from build123d import *

# Parameters (mm, degrees)
F0_R     = 1.75
F1_DEPTH = 1.5


with BuildPart() as f1:
    # F0 (on Right) → F1 (new body)
    with BuildSketch(Plane.YZ):
        Polygon((-3, -1.5), (-3, 0), (3, 0), (3, -1.5), (8, -1.5), (8, 0), (9, 0), (14.459554, 15), (9, 30), (8, 30), (8, 31.5), (3, 31.5), (3, 30), (-3, 30), (-3, 31.5), (-8, 31.5), (-8, 30), (-9, 30), (-3.540446, 15), (-9, 0), (-8, 0), (-8, -1.5), align=None)
        with Locations((0.459554, 15)):
            Circle(F0_R, mode=Mode.SUBTRACT)
    extrude(amount=F1_DEPTH)


solid = f1.part
Geometry: final body of the model. Coordinates: model frame, mm. A direction names the side the tool comes from. Give positions to 0.01 mm unless a question says otherwise; leave off trailing zeros. Write each loop counter-clockwise with the first axis right and the second up, starting at its lowest first coordinate (ties: lowest second). Pieces come first, ordered by that corner, then holes. Notation, with made-up numbers: (84, 47.5) -> (98, 47.5) arc R22 cw to (98, 58.5) -> close; hole circle Ø7 at (9.5, 87). An arc over 180 degrees is marked (long way). Answer as a JSON object with one key per item and string values.
1. Contact query for flat-ended pins moving along their axis: pin 1 (0.8 mm diameter, centred on x = 0.5, y = 0.5, fed in from +Z); pin 2 (0.8 mm diameter, centred on x = 0.5, z = -0.5, fed in from +Y); pin 3 (0.8 mm diameter, centred on x = 1, z = -0.5, fed in from -Y). Output: stop coordinate, or through.
Ans:
{"pin 1": "stops at z = 30", "pin 2": "stops at y = 8", "pin 3": "stops at y = -8"}
2. Ray query, probe 1 along Z at (x, y) = (0.3, 0.5); probe 2 along Z at (x, y) = (0.4, -0.75); probe 3 along Y at (x, z) = (0.8, 28). Return the intervals inside material, ascending. Write a range as from..to.
Ans:
{"probe 1": "z = 0..13.25, 16.75..30", "probe 2": "z = 0..13.74, 16.26..30", "probe 3": "y = -8.27..9.73"}
3. Cut plane A-A on x = 0.55. Output: boundary loops of the cut face in (y, z).
Ans:
{"outline": "(-9, 0) -> (-8, 0) -> (-8, -1.5) -> (-3, -1.5) -> (-3, 0) -> (3, 0) -> (3, -1.5) -> (8, -1.5) -> (8, 0) -> (9, 0) -> (14.46, 15) -> (9, 30) -> (8, 30) -> (8, 31.5) -> (3, 31.5) -> (3, 30) -> (-3, 30) -> (-3, 31.5) -> (-8, 31.5) -> (-8, 30) -> (-9, 30) -> (-3.54, 15) -> close; hole circle Ø3.5 at (0.46, 15)"}
4. Cut plane C-C on z = 1. Output: boundary loops of the cut face in (x, y).
Ans:
{"outline": "(0, -8.64) -> (1.5, -8.64) -> (1.5, 9.36) -> (0, 9.36) -> close"}
5. Mould query, pull axis Y, two halves, no side actions, for faces 1 (the flat face through (0, 3, 15)), 2 (the flat face through (1, -8, -1)), 3 (the flat face through (1, -3, 31)). Classes: pulls with the +Y half, pulls with the -Y half, needs draft (parallel to the pull), parting line crosses it, or undercut.
Ans:
{"face 1": "needs draft", "face 2": "pulls with the -Y half", "face 3": "undercut"}
6. Cut plane B-B on z = 14. Output: boundary loops of the cut face in (x, y).
Ans:
{"outline": "(0, -3.9) -> (1.5, -3.9) -> (1.5, -0.98) -> (0, -0.98) -> close; (0, 1.9) -> (1.5, 1.9) -> (1.5, 14.1) -> (0, 14.1) -> close"}
7. Access query for faces 4 (the flat face through (1, 8, 31)), 5 (the flat face through (1, 3, -1)), 6 (the flat face through (0.74, -6.308, 22.605)), 7 (the flat face through (0.7, -8.5, 0)). Directions: +Z, -Z, +X, -X, +Y, -Y. A direction counts if a zero-diameter tool reaches every point of the face in a straight line with its end or side. Return the directions, or none.
Ans:
{"face 4": "+Z, +X, -X, +Y", "face 5": "-Z, +X, -X", "face 6": "+X, -X, -Y", "face 7": "-Z, +X, -X, -Y"}
